For this review, take the finished solid that the model builds, in its own axes (mm). Round coordinates to 2 decimals unless told otherwise and drop trailing zeros. Write each loop counter-clockwise with the first axis right and the second up, starting at its lowest first coordinate (ties: lowest second). Pieces come first, ordered by that corner, then holes. Notation, with made-up numbers: (-40, 63.25) - (-12, 63.25) arc R33 cw to (-12, 95.25) - close; hole circle Ø6 at (-1.5, 32). An arc over 180 degrees is marked (long way). Answer in a Markdown table with one row per item. Add a question column.
Autodesk Inventor part; units mm, degrees
ref_plane "YZ Plane" through (0, 0, 0) normal (1, 0, 0) x (0, 1, 0)
ref_plane "XZ Plane" through (0, 0, 0) normal (0, 1, 0) x (-1, 0, 0)
ref_plane "XY Plane" through (0, 0, 0) normal (0, 0, 1) x (1, 0, 0)
sketch "スケッチ1" plane through (0, 0, 0) normal (0, 0, 1) x (1, 0, 0)
  circle A0 centre (0, 0) radius 9
  line L0 (-5, 2.8868) -> (5, 2.8868) construction
  line L1 (5, 2.8868) -> (0, -5.7735) construction
  line L2 (0, -5.7735) -> (-5, 2.8868) construction
  circle A1 centre (-5, 2.8868) radius 1.5
  circle A2 centre (5, 2.8868) radius 1.5
  circle A3 centre (0, -5.7735) radius 1.5
  circle A4 centre (0, 4) radius 1.25
  line L3 (0, 0) -> (0, 4) construction
  dimension "d0" = 18
  dimension "d1" = 10
  dimension "d2" = 3
  dimension "d3" = 3
  dimension "d4" = 3
  dimension "d5" = 2.5
  dimension "d6" = 4
extrude "押し出し1" add sketch "スケッチ1" along normal blind 5
chamfer "面取り1" distance 1.75 angle 45 3 edges at (-6.5, 2.8868, 5) (3.5, 2.8868, 5) (-1.5, -5.7735, 5)
properties part number "横回転最終段カム"
Q1. Add section A-A on x = 5. State the section outline as (y, z) points.
Q2. Insertion check: pin 1 Ø5 at (x, y) = (-5, 2.89) entering from +Z; pin 2 Ø2 at (x, z) = (2, 4) entering from +Y; pin 3 Ø4 at (x, y) = (5, 2.89) entering from +Z. Each pin has a flat end and moves straight along its axis. Give the tip position at first contact, or say it passes through.
Q3. To check wall thickness, follow probe 1 along Y at (x, z) = (0, 2); probe 2 along X at (y, z) = (2.25, 4.05); probe 3 along X at (y, z) = (3.5, 4.1). State the ranges of each line that lie inside material, in increasing order.
Q4. Add section C-C on z = 0.5. State the section outline as (x, y) points, then the cut area to 3 significant figures.
Q5. Add section D-D on y = 2. Count the separate pieces of the cut face and the enclosed holes in it, then the cut area to 3 significant figures.
Q6. Add section B-B on x = 0. State the section outline as (y, z) points, then the cut area to 3 significant figures.
Q7. Draft analysis for pull direction Y (two halves, no side actions). For faces 1 (the face through (-5.349, 1.316, 3.359)), 2 (the face through (0, 0, 0)), 3 (the face through (-1.172, -8.923, 2.465)), state which applies: released by +Y, released by -Y, zero draft, split by the parting line, or undercut.
Answer sheet:
| question | item | result |
|---|---|---|
| 1 | outline | (-7.48, 0) - (1.39, 0) - (1.39, 3.25) - (-0.36, 5) - (-7.48, 5) - close; (4.39, 0) - (7.48, 0) - (7.48, 5) - (6.14, 5) - (4.39, 3.25) - close |
| 2 | pin 1 | stops at z = 4.25 |
| 2 | pin 2 | stops at y = 8.94 |
| 2 | pin 3 | stops at z = 3.75 |
| 3 | probe 1 | y = -9 to -7.27, -4.27 to 2.75, 5.25 to 9 |
| 3 | probe 2 | x = -8.71 to -7.21, -2.79 to 2.79, 7.21 to 8.71 |
| 3 | probe 3 | x = -8.29 to -7.27, -2.73 to -1.15, 1.15 to 2.73, 7.27 to 8.29 |
| 4 | outline | circle Ø18 at (0, 0); hole circle Ø3 at (-5, 2.89); hole circle Ø3 at (0, -5.77); hole circle Ø2.5 at (0, 4); hole circle Ø3 at (5, 2.89) |
| 4 | area | 228 mm² |
| 5 | separate pieces | 3 |
| 5 | enclosed holes | 0 |
| 5 | area | 56.7 mm² |
| 6 | outline | (-9, 0) - (-7.27, 0) - (-7.27, 3.25) - (-9, 4.98) - close; (-4.27, 0) - (2.75, 0) - (2.75, 5) - (-2.52, 5) - (-4.27, 3.25) - close; (5.25, 0) - (9, 0) - (9, 5) - (5.25, 5) - close |
| 6 | area | 59.4 mm² |
| 7 | face 1 | undercut |
| 7 | face 2 | zero draft |
| 7 | face 3 | split by the parting line |
